```python
from build123d import *

# Parameters (mm, degrees)
F0_W          = 118.8822906261
F0_H          = 118.8822906261
F1_DEPTH      = 59.441
F1_DEPTH_BACK = 59.441
F3_DEPTH      = 118.883
F4_DEPTH      = 118.883
F5_DEPTH      = 118.883
F6_DEPTH      = 118.883
F8_DEPTH      = 118.8832906261
F9_W          = 22.8022392839
F9_H          = 25.8253251765
F9_H_2        = 1.8863490666
F10_DEPTH     = 118.8832906261


with BuildPart() as f1:
    # F0 (on Front) → F1 (new body, two sides)
    with BuildSketch(Plane.XZ) as f1_sk:
        with Locations((0.0400656936, -7.1052906933)):
            Rectangle(F0_W, F0_H)
    extrude(amount=F1_DEPTH)
    extrude(f1_sk.sketch, amount=-F1_DEPTH_BACK)

    # F2 (on face) → F3 (cut, through all)
    with BuildSketch(Plane.XZ.offset(59.441)):
        with BuildLine():
            Line((59.4812110066, -23.6291363835), (59.4812110066, 3.3540143631))
            Line((59.4812110066, 3.3540143631), (36.171077782, 3.3540143631))
            ThreePointArc((36.171077782, 3.3540143631), (-20.329200251, -16.339702262), (39.0592501624, -23.6291363835))
            Line((39.0592501624, -23.6291363835), (59.4812110066, -23.6291363835))
        make_face()
        with BuildLine():
            ThreePointArc((-59.4010796194, 29.4173564762), (-51.4744086785, 44.6051407739), (-36.1859500408, 52.3358546197))
            Line((-36.1859500408, 52.3358546197), (-59.4010796194, 52.3358546197))
            Line((-59.4010796194, 52.3358546197), (-59.4010796194, 29.4173564762))
        make_face()
    extrude(amount=-F3_DEPTH, mode=Mode.SUBTRACT)

    # F2 (on face) → F4 (cut, through all)
    with BuildSketch(Plane.XZ.offset(59.441)):
        with BuildLine():
            Line((59.4812110066, 52.3358546197), (31.8523161113, 52.3358546197))
            ThreePointArc((31.8523161113, 52.3358546197), (48.2543109443, 47.2441953068), (59.4812110066, 34.2477671802))
            Line((59.4812110066, 34.2477671802), (59.4812110066, 52.3358546197))
        make_face()
    extrude(amount=-F4_DEPTH, mode=Mode.SUBTRACT)

    # F2 (on face) → F5 (cut, through all)
    with BuildSketch(Plane.XZ.offset(59.441)):
        with BuildLine():
            ThreePointArc((-31.8904966116, -66.5464360063), (-47.2927113432, -60.2340029507), (-59.4010796194, -48.8119870424))
            Line((-59.4010796194, -48.8119870424), (-59.4010796194, -66.5464360063))
            Line((-59.4010796194, -66.5464360063), (-31.8904966116, -66.5464360063))
        make_face()
    extrude(amount=-F5_DEPTH, mode=Mode.SUBTRACT)

    # F2 (on face) → F6 (cut, through all)
    with BuildSketch(Plane.XZ.offset(59.441)):
        with BuildLine():
            ThreePointArc((59.4812110066, -47.7445162833), (54.3094541563, -60.4346481438), (42.0443587764, -66.5464360063))
            Line((42.0443587764, -66.5464360063), (59.4812110066, -66.5464360063))
            Line((59.4812110066, -66.5464360063), (59.4812110066, -47.7445162833))
        make_face()
    extrude(amount=-F6_DEPTH, mode=Mode.SUBTRACT)

    # F7 (on face) → F8 (cut, through all)
    with BuildSketch(Plane(origin=(-59.4010796194, 0, 0), x_dir=(0, -1, 0), z_dir=(-1, 0, 0))):
        with BuildLine():
            Line((0, -9.4056399539), (0, -48.8119870424))
            Line((0, -48.8119870424), (59.441, -48.8119870424))
            Line((59.441, -48.8119870424), (59.441, 29.4173564762))
            Line((59.441, 29.4173564762), (30.1632257603, 29.4173564762))
            ThreePointArc((30.1632257603, 29.4173564762), (24.581727157, 2.6248182068), (0, -9.4056399539))
        make_face()
        with BuildLine():
            Line((0, -48.8119870424), (0, -66.7257010937))
            Line((0, -66.7257010937), (59.7706362605, -66.7257010937))
            Line((59.7706362605, -66.7257010937), (59.441, 52.8524406254))
            Line((59.441, 52.8524406254), (0, 52.8524406254))
            ThreePointArc((0, 52.8524406254), (19.098582129, 46.3051274927), (30.1632257603, 29.4173564762))
            Line((30.1632257603, 29.4173564762), (59.441, 29.4173564762))
            Line((59.441, 29.4173564762), (59.441, -48.8119870424))
            Line((59.441, -48.8119870424), (0, -48.8119870424))
        make_face()
        with BuildLine():
            Line((-11.276206805, 29.4173564762), (11.276206805, 29.4173564762))
            ThreePointArc((11.276206805, 29.4173564762), (0, 35.3744003358), (-11.276206805, 29.4173564762))
        make_face()
        with BuildLine():
            ThreePointArc((13.651, 21.7234003358), (13.0437973784, 25.749459321), (11.276206805, 29.4173564762))
            Line((11.276206805, 29.4173564762), (-11.276206805, 29.4173564762))
            ThreePointArc((-11.276206805, 29.4173564762), (-4.0260589852, 8.6796029574), (13.651, 21.7234003358))
        make_face()
    extrude(amount=-F8_DEPTH, mode=Mode.SUBTRACT)

    # F9 (on face) → F10 (cut, through all)
    with BuildSketch(Plane.XY.offset(52.3358546197)):
        with Locations((-0.3479313365, 46.5283374118)):
            Rectangle(F9_W, F9_H)
        with Locations((-0.3479313365, -4.7043729049)):
            Rectangle(F9_W, F9_H_2)
        Polygon((-11.7490509785, -5.6475474382), (-11.7490509785, -48.8955229521), (11.0531883055, -48.660453409), (11.0531883055, -5.6475474382), align=None)
    extrude(amount=-F10_DEPTH, mode=Mode.SUBTRACT)


solid = f1.part
```
The listing builds one solid part. Answer for the finished solid, in the listing's coordinates (mm). A direction names the side the tool comes from. Coordinates: 2 decimals unless noted, no trailing zeros. Write each loop counter-clockwise with the first axis right and the second up, starting at its lowest first coordinate (ties: lowest second). Pieces come first, ordered by that corner, then holes. Notation, with made-up numbers: (54.25, 39) - (83.25, 39) arc R18 ccw to (83.25, 56) - close; hole circle Ø1 at (57.5, 23.25). An arc over 180 degrees is marked (long way). Return JSON: item names as keys, results as strings. Group by question number.
Q1. The part is cut by section A-A on y = 38. Write down the section's boundary in (x, z), and give its area (3 significant figures).
Q2. For a pull along X with two mould halves and no side action, classify faces 4 (the flat face through (11.053, -18, 35)), 5 (the cylindrical face through (-51.65, 23.97, 44.43)), 6 (the cylindrical face through (54.44, 29.3, -60.29)) as +X half, -X half, draft (parallel to the pull), parting line (faces both ways), or undercut.
Q3. Find the intervals of material crossed by line 1 along X through (y, z) = (46.5, 21); line 2 along Y through (x, z) = (46.5, 16); line 3 along Z through (x, y) = (27.5, 29.5), in increasing order. Write a range as [from, to].
Q4. The part is cut by section C-C on x = 16. Write down the section's boundary in (y, z).
Q5. Which of the six approach directions +Z, -Z, +X, -X, +Y, -Y give full straight-line access (tool end or side, diameter ignored) to faces 1 (the flat face through (-1, 0, -44)), 2 (the flat face through (11.053, 46, -55)), 3 (the flat face through (-1, -3.761, 44))?
Q6. The part is cut by section D-D on z = -38. Write down the section's boundary in (x, y), and give its area (3 significant figures).
Q7. The part is cut by section B-B on y = -22.5. Write down the section's boundary in (x, z).
Q8. Flat-ended cylindrical pins translate along their axes: pin 1 Ø20.5 at (y, z) = (40.5, 35) entering from -X; pin 2 Ø19 at (x, z) = (0.5, 40) entering from -Y; pin 3 Ø7 at (x, z) = (-3.5, 32) entering from +Y; pin 4 Ø7 at (y, z) = (40, -52.5) entering from -X. Find the tip coordinate at first contact, or state that the pin passes through.
Evaluation:
{
 "1": {"outline": "(-59.4, -48.81) arc R45.58 ccw to (-31.89, -66.55) - (-11.75, -66.55) - (-11.75, -34.55) arc R30.72 cw to (-11.75, 8.4) - (-11.75, 52.34) - (-36.19, 52.34) arc R28.01 ccw to (-59.4, 29.42) - close; (11.05, -66.55) - (42.04, -66.55) arc R19.41 ccw to (59.48, -47.74) - (59.48, -23.63) - (39.06, -23.63) arc R30.72 cw to (11.05, -43.78) - close; (11.05, 17.64) arc R30.72 cw to (36.17, 3.35) - (59.48, 3.35) - (59.48, 34.25) arc R31.22 ccw to (31.85, 52.34) - (11.05, 52.34) - close", "area": "8,650 mm2"},
 "2": {"face 4": "undercut", "face 5": "-X half", "face 6": "+X half"},
 "3": {"line 1": "x = [-59.4, -11.75], [11.05, 59.48]", "line 2": "y = [-30.6, -12.39], [12.39, 59.44]", "line 3": "z = [-66.55, -38.46], [12.32, 52.34]"},
 "4": {"outline": "(-30.78, 17.1) - (-12.84, 17.1) arc R13.65 cw (long way) to (12.84, 17.1) - (59.44, 17.1) - (59.44, 52.34) - (-5.65, 52.34) arc R31.13 ccw to start; (0, -66.55) - (59.44, -66.55) - (59.44, -43.24) - (0, -43.24) - close"},
 "5": {"face 1": "-Z, +X, -X, -Y", "face 2": "+Z, -Z, +Y", "face 3": "+Z, -Z, -Y"},
 "6": {"outline": "(-59.4, 0) - (-7.73, 0) - (-7.73, 33.62) - (-11.75, 33.62) - (-11.75, 59.44) - (-59.4, 59.44) - close; (28.16, 0) - (59.48, 0) - (59.48, 59.44) - (28.16, 59.44) - close", "area": "4,830 mm2"},
 "7": {"outline": "(-59.4, 0.21) - (-17.48, 0.21) arc R30.72 cw to (-11.75, 8.4) - (-11.75, 43.24) - (-52.77, 43.24) arc R28.01 ccw to (-59.4, 29.42) - close; (11.05, 17.64) arc R30.72 cw to (36.17, 3.35) - (59.48, 3.35) - (59.48, 34.25) arc R31.22 ccw to (53.19, 43.24) - (11.05, 43.24) - close"},
 "8": {"pin 1": "stops at x = -59.4", "pin 2": "stops at y = -3.76", "pin 3": "stops at y = 33.62", "pin 4": "stops at x = -59.26"}
}
